The listing builds one solid part. Answer for the finished solid, in the listing's coordinates (mm). A direction names the side the tool comes from. Give positions to 0.01 mm unless a question says otherwise; leave off trailing zeros. Order: outer loops, then holes, each group sorted by start corner. A loop starts at its lowest first (then second) coordinate and runs counter-clockwise, first axis right, second up. Notation, with made-up numbers: (35, 65.5) -> (71, 65.5) arc R15 cw to (71, 69.5) -> close; hole circle Ø11 at (17.25, 42). An arc over 180 degrees is marked (long way). Write item = value, one per line. Start each with the question number.
```python
from build123d import *

# Parameters (mm, degrees)
SKETCH_5_W          = 80
SKETCH_5_H          = 40
EXTRUDE_3_DEPTH     = 60
DRAFT_6_ANGLE       = -15
DRAFT_7_ANGLE       = -5
SKETCH_8_W          = 35
SKETCH_8_H          = 31.411047216
CUT_EXTRUDE_1_DEPTH = 117


with BuildPart() as part:
    # 스케치5 → 보스-돌출3 (new body)
    with BuildSketch(Plane.XY):
        with Locations((40, 20)):
            Rectangle(SKETCH_5_W, SKETCH_5_H)
    extrude(amount=EXTRUDE_3_DEPTH)

    # 구배6
    draft_6_faces = [part.faces().sort_by_distance(p)[0] for p in [
        (80, 20, 30),
        (0, 20, 30),
    ]]
    draft(draft_6_faces, Plane(origin=(0, 0, 60), x_dir=(0, 0, -1), z_dir=(0, -1, 0)), DRAFT_6_ANGLE)

    # 구배7
    draft_7_faces = [part.faces().sort_by_distance(p)[0] for p in [
        (40, 18.968663077, 0),
        (40, 18.968663077, 60),
    ]]
    draft(draft_7_faces, Plane(origin=(0, 0, 60), x_dir=(0, 0, -1), z_dir=(0, -1, 0)), DRAFT_7_ANGLE)

    # 스케치8 → 컷-돌출1 (cut)
    with BuildSketch(Plane(origin=(0, 0, 0), x_dir=(0, 0, 1), z_dir=(-0.9659258262890682, 0.25881904510252135, 0))):
        with Locations((30, 15.705523608)):
            Rectangle(SKETCH_8_W, SKETCH_8_H)
    extrude(amount=-CUT_EXTRUDE_1_DEPTH, mode=Mode.SUBTRACT)


solid = part.part
```
Item 1: The mould has two halves that part along Z. Classify faces 3 (the flat face through (39.44, 20.28, 58.226)), 4 (the flat face through (39, 0, 6)), 5 (the flat face through (39.44, 20.28, 1.774)), 6 (the flat face through (33, 11, 47.5)): +Z half, -Z half, draft (parallel to the pull), parting line (faces both ways), or undercut.
Item 2: Which of the six approach directions +Z, -Z, +X, -X, +Y, -Y give full straight-line access (tool end or side, diameter ignored) to faces 1 (the flat face through (73.525, 24.164, 29.58)), 2 (the flat face through (41.98, 21.27, 29.76))?
Item 3: Flat-ended cylindrical pins translate along their axes: pin 1 (3 mm diameter, centred on x = 66, y = 11.5, fed in from +Z); pin 2 (2 mm diameter, centred on x = 30, z = 38, fed in from -Y); pin 3 (10 mm diameter, centred on x = 12, y = 30.5, fed in from -Z). Find the tip coordinate at first contact, or state that the pin passes through.
Item 4: A cutting plane is placed at D-D, the plane z = 51.5. Write down the section's boundary in (x, y), plus the area to 3 significant figures.
Item 5: A cutting plane is placed at A-A, the plane y = 9. Write down the section's boundary in (x, z), plus the area to 3 significant figures.
Item 6: A cutting plane is placed at B-B, the plane x = 6.5. Write down the section's boundary in (y, z).
Item 7: Consider L1, parallel to Z at x = 35, y = 10; L2, parallel to Z at x = 73.5, y = 8.5; L3, parallel to X at y = 35, z = 41. Determine where each line is inside the solid, lowest interval first. Write a range as from..to.
Item 8: A cutting plane is placed at C-C, the plane y = 17. Write down the section's boundary in (x, z).
Check values:
q1.face_3 = +Z half
q1.face_4 = draft
q1.face_5 = -Z half
q1.face_6 = undercut
q2.face_1 = +Z, -Z, +X, +Y
q2.face_2 = -X, -Y
q3.pin_1 = 59.13
q3.pin_2 = 24.21
q3.pin_3 = 2.23
q4.outline = (0, 0) -> (80, 0) -> (69.28, 40) -> (10.72, 40) -> close
q4.area = 2,770 mm^2
q5.outline = (2.41, 0.79) -> (77.59, 0.79) -> (77.59, 12.5) -> (2.41, 12.5) -> close; (2.41, 47.5) -> (77.59, 47.5) -> (77.59, 59.21) -> (2.41, 59.21) -> close
q5.area = 1,760 mm^2
q6.outline = (0, 0) -> (24.26, 2.12) -> (24.26, 12.5) -> (0, 12.5) -> close; (0, 47.5) -> (24.26, 47.5) -> (24.26, 57.88) -> (0, 60) -> close
q7.L1 = 0.87..12.5, 47.5..59.13
q7.L2 = 0.74..12.5, 47.5..59.26
q7.L3 = 9.38..70.62
q8.outline = (4.56, 1.49) -> (75.44, 1.49) -> (75.44, 58.51) -> (4.56, 58.51) -> (4.56, 47.5) -> (57.92, 47.5) -> (57.92, 12.5) -> (4.56, 12.5) -> close
